Work out the finished part from the listing and answer in its coordinate system (mm). Face numbers are marked on the shaded views. A direction names the side the tool comes from. Round coordinates to 2 decimals unless told otherwise and drop trailing zeros. Loops run counter-clockwise (first coordinate to the right, second up) from the corner with the lowest first, then second, coordinate; pieces in that order, holes last.
```python
from build123d import *

# Parameters (mm, degrees)
BOSS_EXTRUDE1_DEPTH                                  = 10
SKETCH1_3_R                                          = 11
BOSS_EXTRUDE2_DEPTH                                  = 10
SCHNITT_LINEAR_AUSTRAGEN1_DEPTH                      = 10
STIRNSENKUNG_F_R_M3_ZYLINDERSCHRAUBE_MIT_D           = 2.8
STIRNSENKUNG_F_R_M3_ZYLINDERSCHRAUBE_MIT_DEPTH       = 9.1
STIRNSENKUNG_F_R_M3_ZYLINDERSCHRAUBE_MIT_CBORE_D     = 6.5
STIRNSENKUNG_F_R_M3_ZYLINDERSCHRAUBE_MIT_CBORE_DEPTH = 3.4


with BuildPart() as part:
    # Sketch1 → Boss-Extrude1 (new body)
    with BuildSketch(Plane(origin=(0, 0, 0), x_dir=(1, 0, 0), z_dir=(0, 1, 0))):
        with BuildLine():
            ThreePointArc((-1.081826752, 14.9609375), (-2.92635483, 14.711779206), (-4.72582532, 14.236101118))
            ThreePointArc((-4.72582532, 14.236101118), (-5.548909769, 13.396253221), (-6.724780508, 13.408106769))
            ThreePointArc((-6.724780508, 13.408106769), (-8.333553495, 12.472044185), (-9.814013327, 11.343947391))
            ThreePointArc((-9.814013327, 11.343947391), (-10.253048327, 10.253048327), (-11.343947391, 9.814013327))
            ThreePointArc((-11.343947391, 9.814013327), (-12.472044185, 8.333553495), (-13.408106769, 6.724780508))
            ThreePointArc((-13.408106769, 6.724780508), (-13.396253221, 5.548909769), (-14.236101118, 4.72582532))
            ThreePointArc((-14.236101118, 4.72582532), (-14.711779206, 2.92635483), (-14.9609375, 1.081826752))
            ThreePointArc((-14.9609375, 1.081826752), (-14.5, 0), (-14.9609375, -1.081826752))
            ThreePointArc((-14.9609375, -1.081826752), (-14.711779206, -2.92635483), (-14.236101118, -4.72582532))
            ThreePointArc((-14.236101118, -4.72582532), (-13.396253221, -5.548909769), (-13.408106769, -6.724780508))
            ThreePointArc((-13.408106769, -6.724780508), (-12.472044185, -8.333553495), (-11.343947391, -9.814013327))
            ThreePointArc((-11.343947391, -9.814013327), (-10.253048327, -10.253048327), (-9.814013327, -11.343947391))
            ThreePointArc((-9.814013327, -11.343947391), (-8.333553495, -12.472044185), (-6.724780508, -13.408106769))
            ThreePointArc((-6.724780508, -13.408106769), (-5.548909769, -13.396253221), (-4.72582532, -14.236101118))
            ThreePointArc((-4.72582532, -14.236101118), (-2.92635483, -14.711779206), (-1.081826752, -14.9609375))
            ThreePointArc((-1.081826752, -14.9609375), (0, -14.5), (1.081826752, -14.9609375))
            ThreePointArc((1.081826752, -14.9609375), (2.92635483, -14.711779206), (4.72582532, -14.236101118))
            ThreePointArc((4.72582532, -14.236101118), (5.548909769, -13.396253221), (6.724780508, -13.408106769))
            ThreePointArc((6.724780508, -13.408106769), (8.333553495, -12.472044185), (9.814013327, -11.343947391))
            ThreePointArc((9.814013327, -11.343947391), (10.253048327, -10.253048327), (11.343947391, -9.814013327))
            ThreePointArc((11.343947391, -9.814013327), (12.472044185, -8.333553495), (13.408106769, -6.724780508))
            ThreePointArc((13.408106769, -6.724780508), (13.396253221, -5.548909769), (14.236101118, -4.72582532))
            ThreePointArc((14.236101118, -4.72582532), (14.711779206, -2.92635483), (14.9609375, -1.081826752))
            ThreePointArc((14.9609375, -1.081826752), (14.5, 0), (14.9609375, 1.081826752))
            ThreePointArc((14.9609375, 1.081826752), (14.711779206, 2.92635483), (14.236101118, 4.72582532))
            ThreePointArc((14.236101118, 4.72582532), (13.396253221, 5.548909769), (13.408106769, 6.724780508))
            ThreePointArc((13.408106769, 6.724780508), (12.472044185, 8.333553495), (11.343947391, 9.814013327))
            ThreePointArc((11.343947391, 9.814013327), (10.253048327, 10.253048327), (9.814013327, 11.343947391))
            ThreePointArc((9.814013327, 11.343947391), (8.333553495, 12.472044185), (6.724780508, 13.408106769))
            ThreePointArc((6.724780508, 13.408106769), (5.548909769, 13.396253221), (4.72582532, 14.236101118))
            ThreePointArc((4.72582532, 14.236101118), (2.92635483, 14.711779206), (1.081826752, 14.9609375))
            ThreePointArc((1.081826752, 14.9609375), (0, 14.5), (-1.081826752, 14.9609375))
        make_face()
    extrude(amount=BOSS_EXTRUDE1_DEPTH)

    # Sketch1<3> → Boss-Extrude2 (add)
    with BuildSketch(Plane(origin=(0, 0, 0), x_dir=(1, 0, 0), z_dir=(0, 1, 0))):
        Circle(SKETCH1_3_R)
    extrude(amount=-BOSS_EXTRUDE2_DEPTH)

    # Skizze1 → Schnitt-Linear austragen1 (cut)
    with BuildSketch(Plane.XZ.offset(10)):
        with BuildLine():
            Line((1.9, 2.449489743), (1.9, -2.449489743))
            ThreePointArc((1.9, -2.449489743), (-3.1, 0), (1.9, 2.449489743))
        make_face()
    extrude(amount=-SCHNITT_LINEAR_AUSTRAGEN1_DEPTH, mode=Mode.SUBTRACT)

    # Stirnsenkung für M3 Zylinderschraube mit Innensechskant1
    with Locations(Plane.YZ.offset(11)):
        with Locations((-4.386879559, 0)):
            CounterBoreHole(STIRNSENKUNG_F_R_M3_ZYLINDERSCHRAUBE_MIT_D / 2, STIRNSENKUNG_F_R_M3_ZYLINDERSCHRAUBE_MIT_CBORE_D / 2, STIRNSENKUNG_F_R_M3_ZYLINDERSCHRAUBE_MIT_CBORE_DEPTH, depth=STIRNSENKUNG_F_R_M3_ZYLINDERSCHRAUBE_MIT_DEPTH)


solid = part.part
```
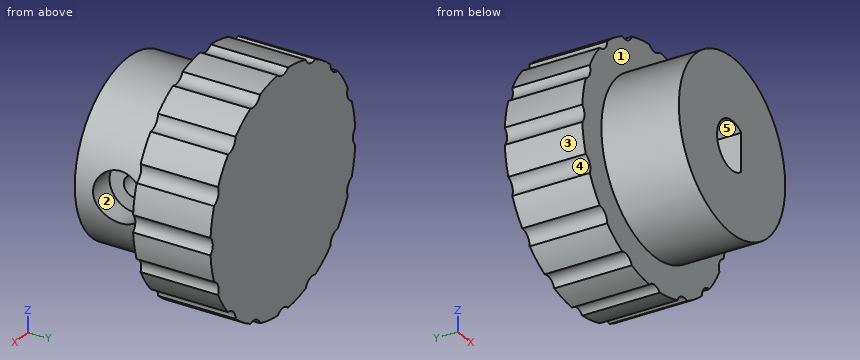
1. Find section C-C (x = 0). Write down the section's boundary in (y, z).
Answer key:
outline: (-10, -11) - (0, -11) - (0, -14.5) - (10, -14.5) - (10, 14.5) - (0, 14.5) - (0, 11) - (-10, 11) - (-10, 3.1) - (0, 3.1) - (0, -3.1) - (-10, -3.1) - close
2. Find section D-D (y = -2.25). Write down the section's boundary in (x, z).
Answer key:
outline: (7.6, -2.45) - (7.6, 2.45) - (10.72, 2.45) arc R11 ccw (long way) to (10.72, -2.45) - close; hole (1.9, -2.45) - (1.9, 2.45) arc R3.1 ccw (long way) to start
3. Find section A-A (z = 0). Write down the section's boundary in (x, y), then the cut area to 3 significant figures.
Answer key:
outline: (-14.5, 0) - (-11, 0) - (-11, -10) - (-3.1, -10) - (-3.1, 0) - (1.9, 0) - (1.9, -2.99) - (7.6, -2.99) - (7.6, -1.14) - (11, -1.14) - (11, 0) - (14.5, 0) - (14.5, 10) - (-14.5, 10) - close; (1.9, -10) - (11, -10) - (11, -7.64) - (7.6, -7.64) - (7.6, -5.79) - (1.9, -5.79) - close
area: 422 mm2
4. Consider probe 1 along Y at (x, z) = (8.4, 0); probe 2 along Z at (x, y) = (0, -5.25); probe 3 along X at (y, z) = (6.5, -11.25). Determine where each line is inside the solid, lowest interval first.
Answer key:
probe 1: y = -10 to -7.64, -1.14 to 10
probe 2: z = -11 to -3.1, 3.1 to 11
probe 3: x = -9.82 to 9.82
5. Determine the mould class of the marked faces 1, 2 and 3 for opening direction Y: +Y half, -Y half, draft (parallel to the pull), parting line (faces both ways), or undercut.
Answer key:
face 1: -Y half
face 2: undercut
face 3: draft
6. Given pin 1 (2.5 mm diameter, centred on y = -4.5, z = -0.5, fed in from -X); pin 2 (1.5 mm diameter, centred on x = -6, y = -5, fed in from +Z); pin 3 (1.5 mm diameter, centred on x = -4, y = -7, fed in from +Z), each flat-ended and moving along its own axis, determine where each tip first touches the part or whether it passes through.
Answer key:
pin 1: stops at x = -11
pin 2: stops at z = 9.67
pin 3: stops at z = 10.51
7. Which of the six approach directions +Z, -Z, +X, -X, +Y, -Y give full straight-line access (tool end or side, diameter ignored) to the marked faces 4 and 5?
Answer key:
face 4: -X, +Y, -Y
face 5: -Y
